from build123d import *

# Parameters (mm, degrees)
F1_DEPTH = 50
F2_DEPTH = 10
F3_R     = 5.5
F4_DEPTH = 10
F5_R     = 6
F6_DEPTH = 12


with BuildPart() as f1:
    # F0 (on Front) → F1 (new body)
    with BuildSketch(Plane.XZ):
        Polygon((-48, 10), (-48, 0), (-18, 0), (-18, 60), (0, 60), (18, 60), (18, 0), (48, 0), (48, 10), (28, 10), (28, 70), (0, 70), (-28, 70), (-28, 10), align=None)
    extrude(amount=F1_DEPTH)

    # F0 (on Front) → F2 (join)
    with BuildSketch(Plane.XZ):
        Polygon((-28, 70), (-48, 10), (-28, 10), align=None)
        Polygon((48, 10), (28, 70), (28, 10), align=None)
        Polygon((-18, 60), (-18, 0), (0, 0), (18, 0), (18, 60), (0, 60), align=None)
    extrude(amount=F2_DEPTH)

    # F3 (on Top) → F4 (cut)
    with BuildSketch(Plane.XY):
        with Locations((-38, -38.325)):
            Circle(F3_R)
        with Locations((38, -38.325)):
            Circle(F3_R)
    extrude(amount=F4_DEPTH, mode=Mode.SUBTRACT)

    # F5 (on face) → F6 (cut)
    with BuildSketch(Plane.XY.offset(70)):
        with Locations((0, -32.725)):
            Circle(F5_R)
    extrude(amount=-F6_DEPTH, mode=Mode.SUBTRACT)


solid = f1.part
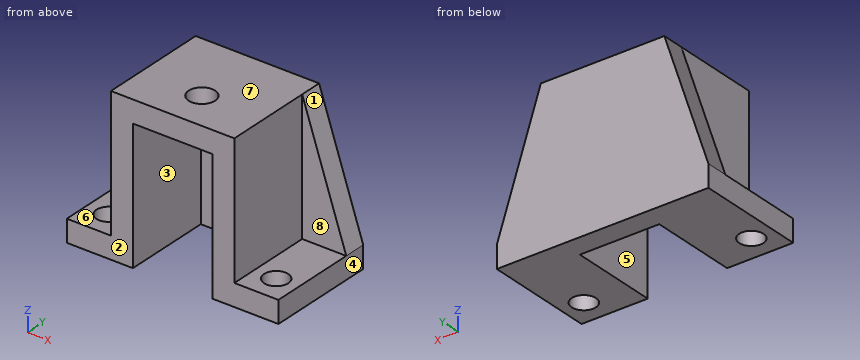
The model under review builds one solid part; all positions refer to its coordinate system, in mm. Face numbers are marked on the shaded views. A direction names the side the tool comes from. Give positions to 0.01 mm unless a question says otherwise; leave off trailing zeros. Write each loop counter-clockwise with the first axis right and the second up, starting at its lowest first coordinate (ties: lowest second). Pieces come first, ordered by that corner, then holes. Notation, with made-up numbers: M -10.75,72 L 36.25,72 A15 cw 36.25,87 Z; hole C 25.25,86 d4. An arc over 180 degrees is marked long. One line per question, with ' | ' between items. Start each with the question number.
Item 1: Wall thickness on line 1 (X direction, y = -33, z = 50); line 2 (Y direction, x = -38, z = 7.5) (3 decimals); line 3 (X direction, y = -36, z = 65): over which ranges is each line inside the solid? List them lowest first. Write a range as from..to.
Item 2: We need section B-B on z = 50.5. Write out the cut boundary in (x, y), plus the area to 3 significant figures.
Item 3: We need section C-C on y = -25.5. Write out the cut boundary in (x, z), plus the area to 3 significant figures.
Item 4: For pin 1 (12.5 mm diameter, centred on x = 38, y = -38.325, fed in from +Z); pin 2 (6 mm diameter, centred on y = -21.5, z = 57.5, fed in from +X); pin 3 (16 mm diameter, centred on x = -38, z = 41.5, fed in from -Y); pin 4 (2 mm diameter, centred on x = 27, z = 24.5, fed in from +Y), all flat-tipped, find the tip position at first contact; note any pin that passes through.
Item 5: We need section D-D on x = 16.5. Write out the cut boundary in (y, z).
Item 6: We need section A-A on x = 0. Write out the cut boundary in (y, z) (3 decimals), plus the area to 3 significant figures.
Item 7: Draft analysis for pull direction X (two halves, no side actions). For the marked faces 1, 2 and 3, state which applies: released by +X, released by -X, zero draft, split by the parting line, or undercut.
Item 8: For the marked faces 4, 5, 6, 7 and 8, list the 3-axis set-ups (+Z, -Z, +X, -X, +Y, -Y) from which the entire face can be reached by the end or side of a thin tool; tool diameter is ignored.
Results found:
1) line 1: x = -28..-18, 18..28 | line 2: y = -50..-43.825, -32.825..0 | line 3: x = -28..-5.03, 5.03..28
2) outline: M -34.5,-10 L -28,-10 L -28,-50 L -18,-50 L -18,-10 L 18,-10 L 18,-50 L 28,-50 L 28,-10 L 34.5,-10 L 34.5,0 L -34.5,0 Z | area: 1,490 mm2
3) outline: M -48,0 L -18,0 L -18,60 L 18,60 L 18,0 L 48,0 L 48,10 L 28,10 L 28,70 L -28,70 L -28,10 L -48,10 Z | area: 2,160 mm2
4) pin 1: stops at z = 10 | pin 2: stops at x = 28 | pin 3: stops at y = -10 | pin 4: stops at y = 0
5) outline: M -50,60 L -10,60 L -10,0 L 0,0 L 0,70 L -50,70 Z
6) outline: M -50,60 L -38.725,60 L -38.725,70 L -50,70 Z; M -26.725,60 L -10,60 L -10,0 L 0,0 L 0,70 L -26.725,70 Z | area: 980 mm2
7) face 1: released by +X | face 2: zero draft | face 3: undercut
8) face 4: +Z, -Z, +X, +Y, -Y | face 5: -Z, -Y | face 6: +Z, -X, -Y | face 7: +Z, +X, -X, +Y, -Y | face 8: +Z, +X, -Y
